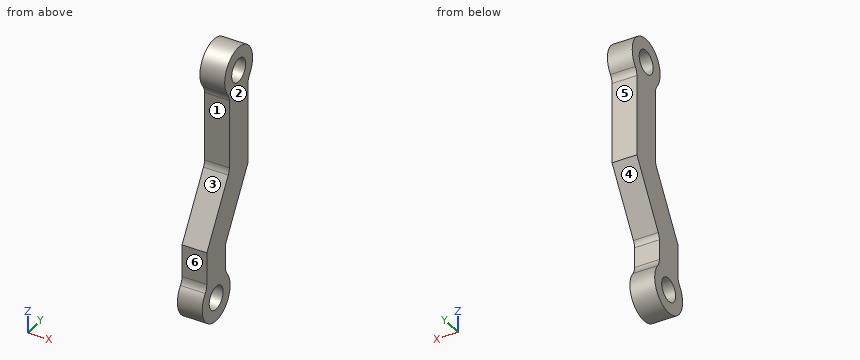
from build123d import *

# Parameters (mm, degrees)
SKETCH2_R           = 1.5
BOSS_EXTRUDE1_DEPTH = 3.175
FILLET1_R           = 1.5875


with BuildPart() as part:
    # Sketch2 → Boss-Extrude1 (new body)
    with BuildSketch(Plane(origin=(0, 0, 0), x_dir=(0, 0, -1), z_dir=(1, 0, 0))):
        with BuildLine():
            Line((13.247387042, 2), (2.236067977, 2))
            ThreePointArc((2.236067977, 2), (-3, 0), (2.236067977, -2))
            Line((2.236067977, -2), (12.13290764, -2))
            Line((12.13290764, -2), (20.13290764, -6.833106971))
            Line((20.13290764, -6.833106971), (24.896839663, -6.833106971))
            ThreePointArc((24.896839663, -6.833106971), (30.13290764, -4.833106971), (24.896839663, -2.833106971))
            Line((24.896839663, -2.833106971), (21.247387042, -2.833106971))
            Line((21.247387042, -2.833106971), (13.247387042, 2))
        make_face()
        Circle(SKETCH2_R, mode=Mode.SUBTRACT)
        with Locations((27.13290764, -4.833106971)):
            Circle(SKETCH2_R, mode=Mode.SUBTRACT)
    extrude(amount=BOSS_EXTRUDE1_DEPTH)

    # Fillet1
    fillet1_edges = [part.edges().sort_by_distance(p)[0] for p in [
        (1.5875, -6.833106971, -24.896839663),
        (1.5875, -2, -12.13290764),
        (1.5875, -2, -2.236067977),
        (1.5875, 2, -2.236067977),
        (1.5875, -2.833106971, -21.247387042),
        (1.5875, -2.833106971, -24.896839663),
    ]]
    fillet(fillet1_edges, radius=FILLET1_R)


solid = part.part
Model file for the job. Use its own axes, mm. Face numbers are marked on the shaded views. A direction names the side the tool comes from. Round coordinates to 2 decimals unless told otherwise and drop trailing zeros. Loops run counter-clockwise (first coordinate to the right, second up) from the corner with the lowest first, then second, coordinate; pieces in that order, holes last. Notation, with made-up numbers: (61, 24.25) - (118, 24.25) arc R25 cw to (118, 60.25) - close; hole circle Ø1 at (33.5, 44.5). An arc over 180 degrees is marked (long way). Write each question's results on one line, items separated by ' | '.
(1) Pin check, flat tips, straight feed: pin 1 (1 mm diameter, centred on x = 0.5, z = -2.5, fed in from +Y); pin 2 (1.6 mm diameter, centred on x = 2, z = -22, fed in from -Y); pin 3 (1 mm diameter, centred on x = 2, z = -7, fed in from -Y). Stop position of each tip, or through.
Answer below:
pin 1: stops at y = 2.25 | pin 2: stops at y = -6.83 | pin 3: stops at y = -2
(2) Saw through at B-B, the plane y = -0.75. List the corners of the cut face in (x, z) (3 decimals).
Answer below:
outline: (0, -17.799) - (3.175, -17.799) - (3.175, -1.299) - (0, -1.299) - close; (0, 1.299) - (3.175, 1.299) - (3.175, 2.905) - (0, 2.905) - close
(3) Saw through at D-D, the plane z = -10. List the corners of the cut face in (x, y) (3 decimals).
Answer below:
outline: (0, -2) - (3.175, -2) - (3.175, 2) - (0, 2) - close
(4) 3-axis set-ups, long thin cutter, end or side, ignore diameter. For the marked faces 3, 4, 5 and 6: which of +Z, -Z, +X, -X, +Y, -Y reach the whole face in a straight line?
Answer below:
face 3: +X, -X, -Y | face 4: +X, -X, +Y | face 5: -Z, +X, -X, +Y | face 6: +Z, +X, -X, -Y
(5) Saw through at A-A, the plane z = 0. List the corners of the cut face in (x, y) (3 decimals), then the cut area to 4 significant figures.
Answer below:
outline: (0, -3) - (3.175, -3) - (3.175, -1.5) - (0, -1.5) - close; (0, 1.5) - (3.175, 1.5) - (3.175, 3) - (0, 3) - close | area: 9.525 mm^2
(6) Wall check: L1, parallel to Y at x = 1.2, z = 0; L2, parallel to Y at x = 2.5, z = -3; L3, parallel to Y at x = 2.15, z = 1. Give the ranges that are in metal, low to high.
Answer below:
L1: y = -3 to -1.5, 1.5 to 3 | L2: y = -2 to 2 | L3: y = -2.83 to -1.12, 1.12 to 2.83
(7) Mould opens along Z. For the marked faces 1 and 2 say: released by +Z, released by -Z, zero draft, split by the parting line, or undercut.
Answer below:
face 1: undercut | face 2: zero draft
(8) Saw through at C-C, the plane x = 1.15. List the corners of the cut face in (y, z) (1 decimal).
Answer below:
outline: (-7.2, -25.3) arc R3 ccw (long way) to (-2.5, -25.3) arc R1.6 cw to (-2.8, -24.3) - (-2.8, -21.7) arc R1.6 cw to (-2.6, -20.9) - (2, -13.2) - (2, -2.9) arc R1.6 cw to (2.3, -1.9) arc R3 ccw (long way) to (-2.3, -1.9) arc R1.6 cw to (-2, -2.9) - (-2, -11.7) arc R1.6 cw to (-2.2, -12.5) - (-6.8, -20.1) - (-6.8, -24.3) arc R1.6 cw to start; hole circle Ø3 at (-4.8, -27.1); hole circle Ø3 at (0, 0)
